Here's how the part is built. I have some questions about the finished solid (model axes, mm). A direction names the side the tool comes from. Coordinates: 2 decimals unless noted, no trailing zeros. Loops run counter-clockwise (first coordinate to the right, second up) from the corner with the lowest first, then second, coordinate; pieces in that order, holes last. Notation, with made-up numbers: (-29, 9) -> (-24, 9) arc R28 cw to (-24, 36) -> close; hole circle Ø1 at (-33.5, -33). An arc over 180 degrees is marked (long way). Answer as a JSON object with one key per item and string values. Group by question number.
1) If we mould it in two halves opening along Y, with no side actions, what happens to faces 1 (the cylindrical face through (-209.23, 1.5, 138.46)), 2 (the flat face through (-204, 21, 74)), 3 (the flat face through (-167, 70, 13))? For each: +Y half, -Y half, draft (parallel to the pull), parting line (faces both ways), or undercut.
2) I want a section at C-C (x = -190). Write out the boundary of the cut face in (y, z), then the cut area to 3 significant figures.
3) I want a section at D-D (y = 13.5). Write out the boundary of the cut face in (x, z), then the cut area to 3 significant figures.
4) I want a section at B-B (y = 0). Count the separate pieces of the cut face and the enclosed holes in it, then the cut area to 3 significant figures.
5) Which directions (+Z, -Z, +X, -X, +Y, -Y) give clear straight access to the entire face, cutting with the end or side of a thin tool? Please do faces 4 (the flat face through (-119, 10, 141)), 5 (the flat face through (-167, 70, 133)), 6 (the flat face through (-116.8, -2.2, 141.5)), 7 (the flat face through (-219, 2, 135.5)), 8 (the cylindrical face through (-160.874, 25.187, 74.101)).
6) I need wall thicknesses on probe 1 along X at (y, z) = (0, 142.95); probe 2 along Y at (x, z) = (-119, 8); probe 3 along Z at (x, y) = (-128, -4.5). Which ranges of each line are inside material? Lowest first, please. Write a range as [from, to].
7) I'm going to push flat-ended pins straight in: pin 1 (5 mm diameter, centred on x = -156, z = 90, fed in from +Y); pin 2 (4 mm diameter, centred on x = -172.5, z = 108.5, fed in from +Y); pin 3 (3.5 mm diameter, centred on x = -214, y = 0, fed in from +Z); pin 4 (3 mm diameter, centred on x = -116, z = 142.5, fed in from +Y). Where does each tip first touch, or does it pass through?
8) I want a section at A-A (x = -214). Write out the boundary of the cut face in (y, z).
```python
from build123d import *

# Parameters (mm, degrees)
SKETCH1_W           = 115
SKETCH1_H           = 20
BOSS_EXTRUDE2_DEPTH = 10
SKETCH5_W           = 75
SKETCH5_H           = 20
BOSS_EXTRUDE3_DEPTH = 62.75
SKETCH6_R           = 5
CUT_EXTRUDE1_DEPTH  = 6
SKETCH7_R           = 2.75
CUT_EXTRUDE2_DEPTH  = 233.838060677
SKETCH8_W           = 75
SKETCH8_H           = 145.5
BOSS_EXTRUDE4_DEPTH = 60


# Read off the part's stored shape, not the designer's step: Cavity1
with BuildPart() as part:
    # Sketch1 → Boss-Extrude2 (new body)
    with BuildSketch(Plane.XY):
        with Locations((-166.5, 0)):
            Rectangle(SKETCH1_W, SKETCH1_H)
    boss_extrude2 = extrude(amount=BOSS_EXTRUDE2_DEPTH)

    # Sketch5 → Boss-Extrude3 (add)
    with BuildSketch(Plane.XY.offset(10)):
        with Locations((-166.5, 0)):
            Rectangle(SKETCH5_W, SKETCH5_H)
    boss_extrude3 = extrude(amount=BOSS_EXTRUDE3_DEPTH)

    # Sketch6 → Cut-Extrude1 (cut)
    with BuildSketch(Plane.XY.offset(10)):
        with Locations((-214, 0)):
            Circle(SKETCH6_R)
        with Locations((-119, 0)):
            Circle(SKETCH6_R)
    cut_extrude1 = extrude(amount=-CUT_EXTRUDE1_DEPTH, mode=Mode.SUBTRACT)

    # Sketch7 → Cut-Extrude2 (cut, through all)
    with BuildSketch(Plane.XY.offset(10)):
        with Locations((-214, 0)):
            Circle(SKETCH7_R)
        with Locations((-119, 0)):
            Circle(SKETCH7_R)
    cut_extrude2 = extrude(amount=-CUT_EXTRUDE2_DEPTH, mode=Mode.SUBTRACT)

    # Mirror2: Boss-Extrude2, Boss-Extrude3, Cut-Extrude1, Cut-Extrude2 across plane
    add(boss_extrude2.mirror(Plane.XY.offset(72.75)))
    add(boss_extrude3.mirror(Plane.XY.offset(72.75)))
    add(cut_extrude1.mirror(Plane.XY.offset(72.75)), mode=Mode.SUBTRACT)
    add(cut_extrude2.mirror(Plane.XY.offset(72.75)), mode=Mode.SUBTRACT)

    # Sketch8 → Boss-Extrude4 (add)
    with BuildSketch(Plane(origin=(0, 10, 0), x_dir=(1, 0, 0), z_dir=(0, 1, 0))):
        with Locations((-166.5, -72.75)):
            Rectangle(SKETCH8_W, SKETCH8_H)
    extrude(amount=BOSS_EXTRUDE4_DEPTH)

    # Cavity1 outline → Cavity1 (revolve, cut)
    with BuildSketch(Plane(origin=(0, 73.114724575, 73.090002845), x_dir=(0, 1, 0), z_dir=(0, 0, -1))):
        with BuildLine():
            add(Edge.make_bspline(
                [(47.94959748, -204), (47.942690938, -201.049048949), (47.938709825, -197.719672316), (47.938508062, -193.954796221)],
                knots=[0.884714855, 0.884714855, 0.884714855, 0.884714855, 0.997011473, 0.997011473, 0.997011473, 0.997011473], degree=3))
            Line((47.938508062, -193.954796221), (47.637, -193.653288159))
            Line((47.637, -193.653288159), (47.9385, -193.653288159))
            Line((47.9385, -193.653288159), (47.9385, -129))
            Line((47.9385, -129), (0, -129))
            Line((0, -129), (0, -204.0000001))
            Line((0, -204.0000001), (47.94959748, -204))
        make_face()
    revolve(axis=Axis((0, 73.114724575, 73.090002845), (1, 0, 0)), mode=Mode.SUBTRACT)


solid = part.part
```
Determined:
{
 "1": {"face 1": "undercut", "face 2": "draft", "face 3": "+Y half"},
 "2": {"outline": "(-10, 0) -> (70, 0) -> (70, 25.25) arc R47.94 cw to (70, 120.93) -> (70, 145.5) -> (-10, 145.5) -> close", "area": "8,330 mm^2"},
 "3": {"outline": "(-204, 0) -> (-129, 0) -> (-129, 145.5) -> (-204, 145.5) -> close", "area": "10,900 mm^2"},
 "4": {"separate pieces": "5", "enclosed holes": "0", "area": "11,400 mm^2"},
 "5": {"face 4": "+Z, -Z, +X, +Y", "face 5": "+Z, -Z, +X, -X, +Y", "face 6": "none", "face 7": "-X, +Y, -Y", "face 8": "+X, +Y"},
 "6": {"probe 1": "[-224, -216.75], [-211.25, -121.75], [-116.25, -109]", "probe 2": "[-10, -5], [5, 10]", "probe 3": "[0, 10], [135.5, 145.5]"},
 "7": {"pin 1": "y = 29.28", "pin 2": "y = 43.14", "pin 3": "through", "pin 4": "y = 10"},
 "8": {"outline": "(-10, 0) -> (-2.75, 0) -> (-2.75, 4) -> (-5, 4) -> (-5, 10) -> (-10, 10) -> close; (-10, 135.5) -> (-5, 135.5) -> (-5, 141.5) -> (-2.75, 141.5) -> (-2.75, 145.5) -> (-10, 145.5) -> close; (2.75, 0) -> (10, 0) -> (10, 10) -> (5, 10) -> (5, 4) -> (2.75, 4) -> close; (2.75, 141.5) -> (5, 141.5) -> (5, 135.5) -> (10, 135.5) -> (10, 145.5) -> (2.75, 145.5) -> close"}
}
